Verification items for the finished model (mm, model axes). Face numbers are marked on the shaded views. A direction names the side the tool comes from. Coordinates: 2 decimals unless noted, no trailing zeros. Order: outer loops, then holes, each group sorted by start corner. A loop starts at its lowest first (then second) coordinate and runs counter-clockwise, first axis right, second up. Notation, with made-up numbers: (44.25, 76.25) -> (64.25, 76.25) arc R9 cw to (64.25, 88.25) -> close; hole circle Ø1 at (52.5, -38). An arc over 180 degrees is marked (long way). Use CSV: the item, a comma, the result in double quotes. Start each with the question number.
1) Sectioned sample at A-A on z = 0. Record the boundary of the cut face in (x, y).
2) Sectioned sample at C-C on x = -19.5. Record the boundary of the cut face in (y, z).
3) Go/stop test with flat-tipped pins: pin 1 (5 mm diameter, centred on y = 15.91, z = 15.91, fed in from +X); pin 2 (9.5 mm diameter, centred on y = -14.5, z = -15.5, fed in from +X); pin 3 (3 mm diameter, centred on x = 0, y = 18.5, fed in from +Z); pin 4 (9.5 mm diameter, centred on y = 15.91, z = -15.91, fed in from -X). Record where each tip stops, or that it passes through.
4) Scan lines: line 1 along X through (y, z) = (2.5, 14); line 2 along X through (y, z) = (0.5, -21); line 3 along Z through (x, y) = (-28.5, -4). Record each from-to range of solid material in increasing order.
5) Tool access check on the marked faces 1 and 2. Record the directions out of +Z, -Z, +X, -X, +Y, -Y that give a thin tool (end or side, any length) a straight path to the whole face; none if there is none.
from build123d import *

# Parameters (mm, degrees)
CHAMFER1_SIZE     = 2
FILLET1_R         = 1
CHAMFER2_SIZE     = 0.5
FILLET2_R         = 1
CHAMFER3_SIZE     = 2
CHAMFER4_SIZE     = 3
HOLE1_D           = 6.5
HOLE1_CBORE_D     = 12
HOLE1_CBORE_DEPTH = 5
CIRPATTERN1_COUNT = 4


with BuildPart() as part:
    # Sketch1 → Revolve1 (revolve)
    with BuildSketch(Plane.XY, mode=Mode.PRIVATE) as revolve1_sk:
        Polygon((-40, 0), (-40, 12.5), (-17.5, 12.5), (-17.5, 15), (0, 15), (0, 30), (10, 30), (10, 0), align=None)
    revolve(revolve1_sk.sketch.rotate(Axis((-40, 0, 0), (1, 0, 0)), 90), axis=Axis((-40, 0, 0), (1, 0, 0)))

    # Chamfer1
    chamfer1_edges = [part.edges().sort_by_distance(p)[0] for p in [
        (-40, 0, -12.5),
    ]]
    chamfer(chamfer1_edges, length=CHAMFER1_SIZE)

    # Fillet1
    fillet1_edges = [part.edges().sort_by_distance(p)[0] for p in [
        (-17.5, 0, -12.5),
    ]]
    fillet(fillet1_edges, radius=FILLET1_R)

    # Chamfer2
    chamfer2_edges = [part.edges().sort_by_distance(p)[0] for p in [
        (-17.5, 0, -15),
    ]]
    chamfer(chamfer2_edges, length=CHAMFER2_SIZE)

    # Fillet2
    fillet2_edges = [part.edges().sort_by_distance(p)[0] for p in [
        (0, 0, -15),
    ]]
    fillet(fillet2_edges, radius=FILLET2_R)

    # Chamfer3
    chamfer3_edges = [part.edges().sort_by_distance(p)[0] for p in [
        (0, 0, -30),
    ]]
    chamfer(chamfer3_edges, length=CHAMFER3_SIZE)

    # Chamfer4
    chamfer4_edges = [part.edges().sort_by_distance(p)[0] for p in [
        (10, 0, -30),
    ]]
    chamfer(chamfer4_edges, length=CHAMFER4_SIZE)

    # Hole1 (through all)
    with Locations(Plane(origin=(10, 0, 0), x_dir=(0, 0, -1), z_dir=(1, 0, 0))):
        with Locations((15.909902577, 15.909902577)):
            hole1 = CounterBoreHole(HOLE1_D / 2, HOLE1_CBORE_D / 2, HOLE1_CBORE_DEPTH)

    # CirPattern1: Hole1 ×4 about axis
    cirpattern1_axis = Axis((0, 0, 0), (1, 0, 0))
    for i in range(1, CIRPATTERN1_COUNT):
        add(hole1.rotate(cirpattern1_axis, i * 360 / CIRPATTERN1_COUNT), mode=Mode.SUBTRACT)

    # Chamfer5: read off the stored shape, not the designer's step
    # Chamfer5: loft between two sections, ruled curve by curve
    chamfer5_from = [
        Edge.make_three_point_arc((8, -21.588647326, 13.972931211), (8, -13.972931211, 10.231157827), (8, -10.231157827, 17.846873942)),
        Edge.make_three_point_arc((8, -10.231157827, 17.846873942), (8, -17.846873942, 21.588647326), (8, -21.588647326, 13.972931211)),
    ]
    chamfer5_to = [
        Edge.make_three_point_arc((10.000000095, -23.481562332, 13.327274059), (10.000000095, -13.327274059, 8.338242821), (10.000000095, -8.338242821, 18.492531095)),
        Edge.make_three_point_arc((10.000000095, -8.338242821, 18.492531095), (10.000000095, -18.492531095, 23.481562332), (10.000000095, -23.481562332, 13.327274059)),
    ]
    chamfer5 = Solid(Shell([*[Face.make_surface_from_curves(chamfer5_from[k], chamfer5_to[k]) for k in range(2)], Face(Wire(chamfer5_from)), Face(Wire(chamfer5_to))]))
    add(chamfer5, mode=Mode.SUBTRACT)

    # Chamfer5 2: loft between two sections, ruled curve by curve
    chamfer5_2_from = [
        Edge.make_three_point_arc((8, -13.972931211, -21.588647326), (8, -10.231157827, -13.972931211), (8, -17.846873942, -10.231157827)),
        Edge.make_three_point_arc((8, -17.846873942, -10.231157827), (8, -21.588647326, -17.846873942), (8, -13.972931211, -21.588647326)),
    ]
    chamfer5_2_to = [
        Edge.make_three_point_arc((10.000000095, -13.327274059, -23.481562332), (10.000000095, -8.338242821, -13.327274059), (10.000000095, -18.492531095, -8.338242821)),
        Edge.make_three_point_arc((10.000000095, -18.492531095, -8.338242821), (10.000000095, -23.481562332, -18.492531095), (10.000000095, -13.327274059, -23.481562332)),
    ]
    chamfer5_2 = Solid(Shell([*[Face.make_surface_from_curves(chamfer5_2_from[k], chamfer5_2_to[k]) for k in range(2)], Face(Wire(chamfer5_2_from)), Face(Wire(chamfer5_2_to))]))
    add(chamfer5_2, mode=Mode.SUBTRACT)

    # Chamfer5 3: loft between two sections, ruled curve by curve
    chamfer5_3_from = [
        Edge.make_three_point_arc((8, 21.588647326, -13.972931211), (8, 13.972931211, -10.231157827), (8, 10.231157827, -17.846873942)),
        Edge.make_three_point_arc((8, 10.231157827, -17.846873942), (8, 17.846873942, -21.588647326), (8, 21.588647326, -13.972931211)),
    ]
    chamfer5_3_to = [
        Edge.make_three_point_arc((10.000000095, 23.481562332, -13.327274059), (10.000000095, 13.327274059, -8.338242821), (10.000000095, 8.338242821, -18.492531095)),
        Edge.make_three_point_arc((10.000000095, 8.338242821, -18.492531095), (10.000000095, 18.492531095, -23.481562332), (10.000000095, 23.481562332, -13.327274059)),
    ]
    chamfer5_3 = Solid(Shell([*[Face.make_surface_from_curves(chamfer5_3_from[k], chamfer5_3_to[k]) for k in range(2)], Face(Wire(chamfer5_3_from)), Face(Wire(chamfer5_3_to))]))
    add(chamfer5_3, mode=Mode.SUBTRACT)

    # Chamfer5 4: loft between two sections, ruled curve by curve
    chamfer5_4_from = [
        Edge.make_three_point_arc((8, 13.972931211, 21.588647326), (8, 10.231157827, 13.972931211), (8, 17.846873942, 10.231157827)),
        Edge.make_three_point_arc((8, 17.846873942, 10.231157827), (8, 21.588647326, 17.846873942), (8, 13.972931211, 21.588647326)),
    ]
    chamfer5_4_to = [
        Edge.make_three_point_arc((10.000000095, 13.327274059, 23.481562332), (10.000000095, 8.338242821, 13.327274059), (10.000000095, 18.492531095, 8.338242821)),
        Edge.make_three_point_arc((10.000000095, 18.492531095, 8.338242821), (10.000000095, 23.481562332, 18.492531095), (10.000000095, 13.327274059, 23.481562332)),
    ]
    chamfer5_4 = Solid(Shell([*[Face.make_surface_from_curves(chamfer5_4_from[k], chamfer5_4_to[k]) for k in range(2)], Face(Wire(chamfer5_4_from)), Face(Wire(chamfer5_4_to))]))
    add(chamfer5_4, mode=Mode.SUBTRACT)


solid = part.part
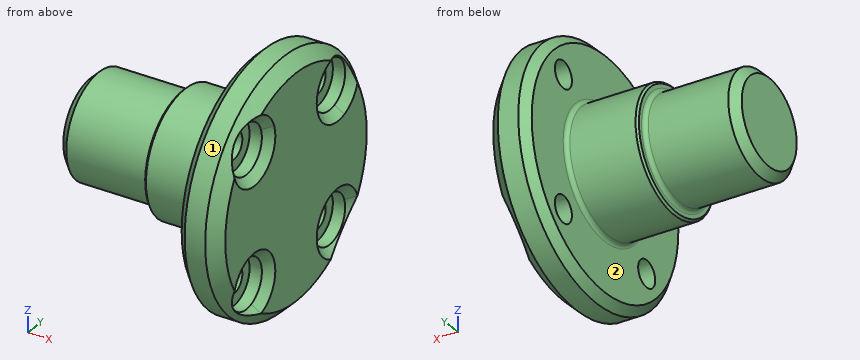
Answers follow:
1,outline,"(-40, -10.5) -> (-38, -12.5) -> (-18.5, -12.5) arc R1 cw to (-17.5, -13.5) -> (-17.5, -14.5) -> (-17, -15) -> (-1, -15) arc R1 cw to (0, -16) -> (0, -28) -> (2, -30) -> (7, -30) -> (10, -27) -> (10, 27) -> (7, 30) -> (2, 30) -> (0, 28) -> (0, 16) arc R1 cw to (-1, 15) -> (-17, 15) -> (-17.5, 14.5) -> (-17.5, 13.5) arc R1 cw to (-18.5, 12.5) -> (-38, 12.5) -> (-40, 10.5) -> close"
2,outline,"circle Ø25 at (0, 0)"
3,pin 1,"passes through"
3,pin 2,"stops at x = 8.22"
3,pin 3,"stops at z = 23.31"
3,pin 4,"stops at x = 0"
4,line 1,"x = -17.5 to 10"
4,line 2,"x = 0 to 10"
4,line 3,"z = -11.84 to 11.84"
5,face 1,"+X, -X"
5,face 2,"-X"
